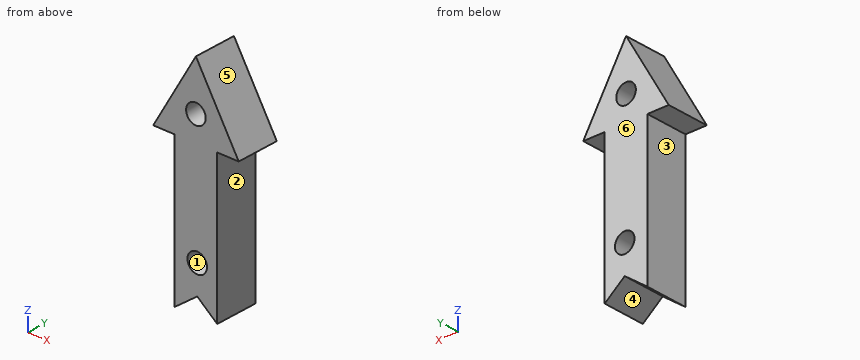
from build123d import *

# Parameters (mm, degrees)
F0_R     = 4.365625
F1_DEPTH = 19.05


with BuildPart() as f1:
    # F0 (on Front) → F1 (new body)
    with BuildSketch(Plane.XZ):
        with BuildLine():
            ThreePointArc((-4.968861, 51.842821), (-0.603236, 56.208446), (3.762389, 51.842821))
            Line((3.762389, 51.842821), (8.921764, 51.842821))
            Line((8.921764, 51.842821), (8.921764, 40.727447))
            Line((8.921764, 40.727447), (18.526586, 40.751948))
            Line((18.526586, 40.751948), (-0.603236, 73.701302))
            Line((-0.603236, 73.701302), (-19.653236, 40.654553))
            Line((-19.653236, 40.654553), (-10.128236, 40.678851))
            Line((-10.128236, 40.678851), (-10.128236, 51.842821))
            Line((-10.128236, 51.842821), (-4.968861, 51.842821))
        make_face()
        Polygon((8.921764, -24.357179), (8.921764, 40.727447), (-10.128236, 40.678851), (-10.128236, -24.804613), (0, -17.142445), align=None)
        with Locations((0, -4.442445)):
            Circle(F0_R, mode=Mode.SUBTRACT)
        with BuildLine():
            Line((8.921764, 51.842821), (3.762389, 51.842821))
            ThreePointArc((3.762389, 51.842821), (-0.603236, 47.477196), (-4.968861, 51.842821))
            Line((-4.968861, 51.842821), (-10.128236, 51.842821))
            Line((-10.128236, 51.842821), (-10.128236, 40.678851))
            Line((-10.128236, 40.678851), (8.921764, 40.727447))
            Line((8.921764, 40.727447), (8.921764, 51.842821))
        make_face()
    extrude(amount=F1_DEPTH)


solid = f1.part
Can you work these out from the model? Positions are in its coordinate system, mm. Face numbers are marked on the shaded views. A direction names the side the tool comes from. Round coordinates to 2 decimals unless told otherwise and drop trailing zeros. Write each loop counter-clockwise with the first axis right and the second up, starting at its lowest first coordinate (ties: lowest second). Pieces come first, ordered by that corner, then holes. Notation, with made-up numbers: M 38,-18.5 L 73,-18.5 A11 cw 73,-4.5 Z; hole C -22.75,-34.75 d8. An arc over 180 degrees is marked long. Use a Markdown table: item, result.
Item 1: We'd pull the mould along X, two halves only. Please class the marked faces 3, 4, 5 and 6: released by +X, released by -X, zero draft, split by the parting line, or undercut.
Found:
| item | result |
|---|---|
| face 3 | released by -X |
| face 4 | undercut |
| face 5 | released by +X |
| face 6 | zero draft |
Item 2: I want a section at C-C (z = 33). List the corners of the cut face in (x, y) for me, and give its area (3 significant figures).
Found:
| item | result |
|---|---|
| outline | M -10.13,-19.05 L 8.92,-19.05 L 8.92,0 L -10.13,0 Z |
| area | 363 mm2 |
Item 3: I want a section at B-B (y = -2.5). List the corners of the cut face in (x, z) for me.
Found:
| item | result |
|---|---|
| outline | M -19.65,40.65 L -10.13,40.68 L -10.13,-24.8 L 0,-17.14 L 8.92,-24.36 L 8.92,40.73 L 18.53,40.75 L -0.6,73.7 Z; hole C -0.6,51.84 d8.73; hole C 0,-4.44 d8.73 |
Item 4: For pin 1 Ø4 at (x, z) = (5.5, 2.5) entering from +Y; pin 2 Ø3 at (y, z) = (-16, 47) entering from +X; pin 3 Ø1.5 at (y, z) = (-11.5, 34.5) entering from -X; pin 4 Ø7 at (x, z) = (0, -4.44) entering from +Y, each with a flat end and sliding along its axis, tell me the tip position at first contact or that it passes through.
Found:
| item | result |
|---|---|
| pin 1 | stops at y = 0 |
| pin 2 | stops at x = 15.77 |
| pin 3 | stops at x = -10.13 |
| pin 4 | passes through |
Item 5: I want a section at A-A (x = -2). List the corners of the cut face in (y, z) for me.
Found:
| item | result |
|---|---|
| outline | M -19.05,-18.66 L 0,-18.66 L 0,-8.32 L -19.05,-8.32 Z; M -19.05,-0.56 L 0,-0.56 L 0,47.71 L -19.05,47.71 Z; M -19.05,55.98 L 0,55.98 L 0,71.28 L -19.05,71.28 Z |
Item 6: If I drill on line 1 along Z through (x, y) = (0, -11.25); line 2 along Z through (x, y) = (-3, -10.25); line 3 along X through (y, z) = (-1.5, 10), over which ranges is the centre line in solid material (lowest first)? Write a range as [from, to].
Found:
| item | result |
|---|---|
| line 1 | z = [-17.14, -8.81], [-0.08, 47.52], [56.17, 72.66] |
| line 2 | z = [-19.41, -7.61], [-1.27, 48.19], [55.49, 69.54] |
| line 3 | x = [-10.13, 8.92] |
Item 7: Which directions (+Z, -Z, +X, -X, +Y, -Y) give clear straight access to the entire face, cutting with the end or side of a thin tool? Please do the marked faces 1 and 2.
Found:
| item | result |
|---|---|
| face 1 | +Y, -Y |
| face 2 | -Z, +X, +Y, -Y |
Item 8: I want a section at D-D (x = 2). List the corners of the cut face in (y, z) for me.
Found:
| item | result |
|---|---|
| outline | M -19.05,-18.76 L 0,-18.76 L 0,-8.32 L -19.05,-8.32 Z; M -19.05,-0.56 L 0,-0.56 L 0,48.34 L -19.05,48.34 Z; M -19.05,55.35 L 0,55.35 L 0,69.22 L -19.05,69.22 Z |
